```python
from build123d import *

# Parameters (mm, degrees)
SKETCH_W     = 31.8
SKETCH_H     = 13
PAD_DEPTH    = 3
SKETCH001_W  = 9
SKETCH001_H  = 6.5
PAD001_DEPTH = 10
SKETCH002_W  = 5
SKETCH002_H  = 13
PAD002_DEPTH = 15
PAD002_TAPER = 0.5
POCKET_DEPTH = 28.001
FILLET_R     = 3.5
FILLET001_R  = 1


with BuildPart() as part:
    # Sketch → Pad (new body)
    with BuildSketch(Plane.XZ):
        Rectangle(SKETCH_W, SKETCH_H)
    extrude(amount=PAD_DEPTH)

    # Sketch001 (on Face6 of Pad) → Pad001 (join)
    with BuildSketch(Plane.XZ.offset(3)):
        with Locations((-9.5, 0)):
            Rectangle(SKETCH001_W, SKETCH001_H)
        with Locations((9.5, 0)):
            Rectangle(SKETCH001_W, SKETCH001_H)
    extrude(amount=PAD001_DEPTH)

    # Sketch002 (on Face4 of Pad001) → Pad002 (join)
    with BuildSketch(Plane(origin=(0, 0, 0), x_dir=(1, 0, 0), z_dir=(0, 1, 0))):
        Rectangle(SKETCH002_W, SKETCH002_H)
    extrude(amount=PAD002_DEPTH, taper=PAD002_TAPER)

    # Sketch003 (on Face10 of Pad002) → Pocket (cut, through all)
    with BuildSketch(Plane(origin=(0, 15, 0), x_dir=(1, 0, 0), z_dir=(0, 1, 0))):
        Polygon((-0.625, -4), (0.625, -4), (0.625, -3), (0.5, -3), (0.5, -2), (0.625, -2), (0.625, 2), (0.5, 2), (0.5, 3), (0.625, 3), (0.625, 4), (-0.625, 4), (-0.625, 3), (-0.499997, 3), (-0.5, 2), (-0.625, 2), (-0.625, -2), (-0.5, -2), (-0.5, -3), (-0.625, -3), align=None)
    extrude(amount=-POCKET_DEPTH, mode=Mode.SUBTRACT)

    # Fillet
    fillet_edges = [part.edges().sort_by_distance(p)[0] for p in [
        (15.9, -1.5, -6.5),
        (-15.9, -1.5, -6.5),
        (-15.9, -1.5, 6.5),
        (15.9, -1.5, 6.5),
    ]]
    fillet(fillet_edges, radius=FILLET_R)

    # Fillet001
    fillet001_edges = [part.edges().sort_by_distance(p)[0] for p in [
        (-14, -8, -3.25),
        (-14, -8, 3.25),
        (-5, -8, -3.25),
        (5, -8, -3.25),
        (14, -8, -3.25),
        (-5, -8, 3.25),
        (5, -8, 3.25),
        (14, -8, 3.25),
    ]]
    fillet(fillet001_edges, radius=FILLET001_R)


solid = part.part
```
Read the model definition and answer for the solid it produces. Units are mm, in the model's axes. A direction names the side the tool comes from. Coordinates: 2 decimals unless noted, no trailing zeros. Order: outer loops, then holes, each group sorted by start corner. A loop starts at its lowest first (then second) coordinate and runs counter-clockwise, first axis right, second up. Notation, with made-up numbers: (-14.75, 7) - (3.25, 7) arc R17 ccw to (3.25, 17) - close; hole circle Ø5 at (54.25, -38.75). An arc over 180 degrees is marked (long way). Answer as a JSON object with one key per item and string values. Group by question number.
Item 1: Section A-A (y = -6.75) is taken. Give the vertices of the cut face in (x, z), plus the area to 3 significant figures.
Item 2: Consider probe 1 along Y at (x, z) = (0, 4.5); probe 2 along Z at (x, y) = (-6, -10); probe 3 along Y at (x, z) = (7.5, -3.75). Determine where each line is inside the solid, lowest interval first. Write a range as from..to.
Item 3: Section C-C (x = -5.5) is taken. Give the vertices of the cut face in (y, z), plus the area to 3 significant figures.
Item 4: A tool of negligible diameter and unlimited length cuts with its end or side. For faces 1 (the face through (-14, -8, 0)), 2 (the face through (-5.301, -8.07, -2.965)), 3 (the face through (5.285, -8.07, 2.949)), 4 (the face through (0, 6, -4)), 5 (the face through (9, -8, 3.25)), from which of +Z, -Z, +X, -X, +Y, -Y can it reach the whole face along a straight path? Write none if from no direction.
Item 5: Section B-B (x = 14.5) is taken. Give the vertices of the cut face in (y, z).
Item 6: Flat-ended cylindrical pins translate along their axes: P1, Ø2, axis at x = 12, z = 5, coming from the +Y side; P2, Ø2, axis at x = -2, z = 2, coming from the -Y side; P3, Ø0.8, axis at y = 8.5, z = 3.5, coming from the -X side. Find the tip coordinate at first contact, or state that the pin passes through.
Item 7: Section D-D (x = 3) is taken. Give the vertices of the cut face in (y, z).
Results are:
{
 "1": {"outline": "(-14, -2.25) arc R1 ccw to (-13, -3.25) - (-6, -3.25) arc R1 ccw to (-5, -2.25) - (-5, 2.25) arc R1 ccw to (-6, 3.25) - (-13, 3.25) arc R1 ccw to (-14, 2.25) - close; (5, -2.25) arc R1 ccw to (6, -3.25) - (13, -3.25) arc R1 ccw to (14, -2.25) - (14, 2.25) arc R1 ccw to (13, 3.25) - (6, 3.25) arc R1 ccw to (5, 2.25) - close", "area": "115 mm^2"},
 "2": {"probe 1": "y = -3..15", "probe 2": "z = -3.25..3.25", "probe 3": "y = -3..0"},
 "3": {"outline": "(-13, -3.12) - (-3, -3.12) - (-3, -6.5) - (0, -6.5) - (0, 6.5) - (-3, 6.5) - (-3, 3.12) - (-13, 3.12) - close", "area": "101 mm^2"},
 "4": {"face 1": "+Z, -Z, -X, -Y", "face 2": "-Z, -Y", "face 3": "+Z, -Y", "face 4": "+Y, -Y", "face 5": "+Z, +X, -X, -Y"},
 "5": {"outline": "(-3, -5.8) - (0, -5.8) - (0, 5.8) - (-3, 5.8) - close"},
 "6": {"P1": "stops at y = 0", "P2": "stops at y = -3", "P3": "stops at x = -2.43"},
 "7": {"outline": "(-3, -6.5) - (0, -6.5) - (0, 6.5) - (-3, 6.5) - close"}
}
